Source: CAD feature listing. Evaluate the final solid. Frame: model axes, mm. Give positions to 0.01 mm unless a question says otherwise; leave off trailing zeros. Loops run counter-clockwise (first coordinate to the right, second up) from the corner with the lowest first, then second, coordinate; pieces in that order, holes last. Notation, with made-up numbers: (-17.75, 1.5) - (-10.75, 1.5) arc R38 ccw to (-10.75, 39.5) - close; hole circle Ø7 at (50, 58.5). An arc over 180 degrees is marked (long way). Write each question's results on one line, items separated by ' | '. Start each with the question number.
(1) Material intervals for line 1 along X through (y, z) = (-2.9, 25); line 2 along Y through (x, z) = (5, 26); line 3 along X through (y, z) = (1.6, -175), sorted ascending. Write a range as [from, to].
(2) Contact query for a flat-ended pin moving along its axis: pin 1 (4.5 mm diameter, centred on x = 0, z = -50, fed in from +Y). Output: stop coordinate, or through.
(3) Cut plane A-A on z = -40.5. Return the cut outline in (x, y), then the cut area to 3 significant figures.
from build123d import *

# Parameters (mm, degrees)
SKETCH_1_W                = 12
SKETCH_1_H                = 8
EXTRUDE_1_DEPTH           = 225
CUT_EXTRUDE_1_DEPTH       = 451
CHAMFER_1_SIZE            = 0.5
HOLE_WIZARD_3_D           = 3.4
HOLE_WIZARD_3_CBORE_D     = 6
HOLE_WIZARD_3_CBORE_DEPTH = 3.4


with BuildPart() as part:
    # 草图1 → 凸台-拉伸1 (new body, symmetric)
    with BuildSketch(Plane.XY):
        Rectangle(SKETCH_1_W, SKETCH_1_H)
    extrude(amount=EXTRUDE_1_DEPTH, both=True)

    # 草图2 → 切除-拉伸1 (cut, through all)
    with BuildSketch(Plane(origin=(0, 0, -225), x_dir=(-1, 0, 0), z_dir=(0, 0, -1))):
        Polygon((5.2, 2.6), (4.8, 2.6), (4.8, 1.4), (5.2, 1.4), (6, 1), (6, 3), align=None)
    cut_extrude_1 = extrude(amount=-CUT_EXTRUDE_1_DEPTH, mode=Mode.SUBTRACT)

    # 镜向1: 切除-拉伸1 across plane
    add(cut_extrude_1.mirror(Plane(origin=(0, 0, 0), x_dir=(0, 0, 1), z_dir=(1, 0, 0))), mode=Mode.SUBTRACT)

    # 倒角1
    chamfer_1_edges = [part.edges().sort_by_distance(p)[0] for p in [
        (6, -4, 0),
        (-6, -4, 0),
        (-6, 4, 0),
        (6, 4, 0),
    ]]
    chamfer(chamfer_1_edges, length=CHAMFER_1_SIZE)

    # 打孔尺寸(%根据)内六角圆柱头螺钉的类型3 (through all)
    with Locations(Plane(origin=(0, 4, 0), x_dir=(1, 0, 0), z_dir=(0, 1, 0))):
        with Locations((0, 125), (0, 100), (0, 75), (0, 50), (0, 25), (0, 0), (0, -25), (0, -50), (0, -75), (0, -100), (0, -125), (0, 150), (0, 175), (0, 200), (0, -150), (0, -175), (0, -200), (0, -225), (0, 225)):
            CounterBoreHole(HOLE_WIZARD_3_D / 2, HOLE_WIZARD_3_CBORE_D / 2, HOLE_WIZARD_3_CBORE_DEPTH)


solid = part.part
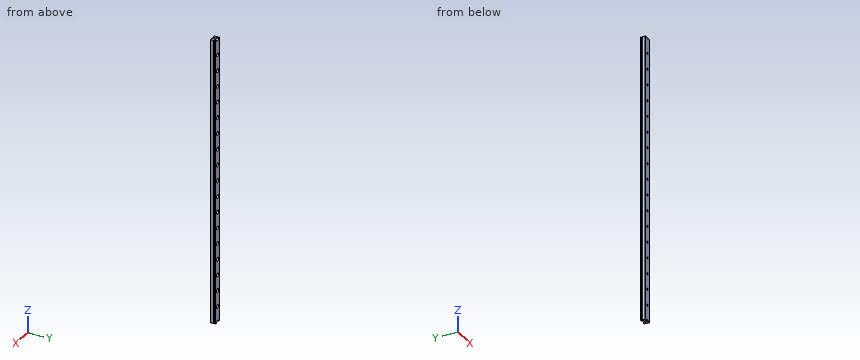
Ans:
1) line 1: [-6, -1.7], [1.7, 6] | line 2: [-4, 1.4], [2.6, 4] | line 3: [-4.8, -3], [3, 4.8]
2) pin 1: y = 0.6
3) outline: (-6, -3.5) - (-5.5, -4) - (5.5, -4) - (6, -3.5) - (6, 1) - (5.2, 1.4) - (4.8, 1.4) - (4.8, 2.6) - (5.2, 2.6) - (6, 3) - (6, 3.5) - (5.5, 4) - (-5.5, 4) - (-6, 3.5) - (-6, 3) - (-5.2, 2.6) - (-4.8, 2.6) - (-4.8, 1.4) - (-5.2, 1.4) - (-6, 1) - close | area: 92.0 mm^2
